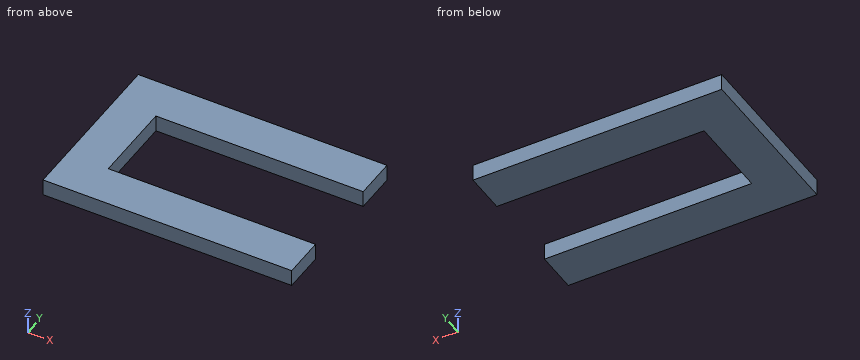
```python
from build123d import *

# Parameters (mm, degrees)
BOSS_EXTRUDE1_DEPTH = 2


with BuildPart() as part:
    # Sketch1 → Boss-Extrude1 (new body)
    with BuildSketch(Plane.XY):
        Polygon((-15, 10), (-15, 0), (-10, 0), (-10, 5), (7.5, 5), (15, 10), align=None)
        Polygon((-7.5, -5), (-15, -10), (15, -10), (15, -5), align=None)
        Polygon((15, 10), (7.5, 5), (15, 5), align=None)
        Polygon((-15, 0), (-15, -10), (-7.5, -5), (-10, -5), (-10, 0), align=None)
    extrude(amount=BOSS_EXTRUDE1_DEPTH)


solid = part.part
```
Design review of the part built by this model. Coordinates are the model's own, in mm. Round coordinates to 2 decimals unless told otherwise and drop trailing zeros. Order: outer loops, then holes, each group sorted by start corner. A loop starts at its lowest first (then second) coordinate and runs counter-clockwise, first axis right, second up. Notation, with made-up numbers: (-37.5, 63) - (-9.5, 63) arc R13 ccw to (-9.5, 84) - close; hole circle Ø6 at (44, -23.5). An arc over 180 degrees is marked (long way). Return JSON: item names as keys, results as strings.
Q1. Consider section A-A on x = -1.5. Write out the cut boundary in (y, z).
Computed values:
{"outline": "(-10, 0) - (-5, 0) - (-5, 2) - (-10, 2) - close; (5, 0) - (10, 0) - (10, 2) - (5, 2) - close"}
Q2. Wall thickness on L1, parallel to Y at x = 5.5, z = 0.6; L2, parallel to X at y = 4.5, z = 0.45: over which ranges is each line inside the solid? List them lowest first. Write a range as [from, to].
Computed values:
{"L1": "y = [-10, -5], [5, 10]", "L2": "x = [-15, -10]"}
Q3. Consider section B-B on z = 0.8. Write out the cut boundary in (x, y), plus the area to 3 significant figures.
Computed values:
{"outline": "(-15, -10) - (15, -10) - (15, -5) - (-10, -5) - (-10, 5) - (15, 5) - (15, 10) - (-15, 10) - close", "area": "350 mm2"}
Q4. Consider section C-C on y = 2.5. Write out the cut boundary in (x, z).
Computed values:
{"outline": "(-15, 0) - (-10, 0) - (-10, 2) - (-15, 2) - close"}
